Build history of the part. All positions in model axes, mm. A direction names the side the tool comes from. Round coordinates to 2 decimals unless told otherwise and drop trailing zeros. Write each loop counter-clockwise with the first axis right and the second up, starting at its lowest first coordinate (ties: lowest second). Pieces come first, ordered by that corner, then holes. Notation, with made-up numbers: (41.5, 34.5) -> (45.5, 34.5) arc R25 ccw to (45.5, 67.5) -> close; hole circle Ø11 at (-39, -12.5). An arc over 180 degrees is marked (long way). Return JSON: item names as keys, results as strings.
from build123d import *

# Parameters (mm, degrees)
F0_R     = 3
F1_DEPTH = 5
F0_R_2   = 1.6
F2_DEPTH = 2
F4_W     = 30
F4_H     = 20
F5_DEPTH = 2
F6_R     = 0.99999


# Not quite as in the source:
# - a fillet or chamfer is up to 0.001 mm smaller than in the source, because OpenCascade refuses the exact size


with BuildPart() as f1:
    # F0 (on Top) → F1 (new body)
    with BuildSketch(Plane.XY):
        with BuildLine():
            Line((-47.4, -10), (0, -10))
            ThreePointArc((0, -10), (10, 0), (0, 10))
            Line((0, 10), (-47.4, 10))
            ThreePointArc((-47.4, 10), (-57.4, 0), (-47.4, -10))
        make_face()
        with Locations((-47.4, 0)):
            Circle(F0_R, mode=Mode.SUBTRACT)
        Polygon((-6.5240580418, 0), (-3.2620290209, 5.65), (3.2620290209, 5.65), (6.5240580418, 0), (3.2620290209, -5.65), (-3.2620290209, -5.65), align=None, mode=Mode.SUBTRACT)
    extrude(amount=F1_DEPTH)

    # F0 (on Top) → F2 (join)
    with BuildSketch(Plane.XY):
        Polygon((3.2620290209, 5.65), (-3.2620290209, 5.65), (-6.5240580418, 0), (-3.2620290209, -5.65), (3.2620290209, -5.65), (6.5240580418, 0), align=None)
        Circle(F0_R_2, mode=Mode.SUBTRACT)
    extrude(amount=F2_DEPTH)

    # F4 (on face) → F5 (cut)
    with BuildSketch(Plane(origin=(0, 0, 0), x_dir=(1, 0, 0), z_dir=(0, 0, -1))):
        with Locations((-44.4, 0)):
            Rectangle(F4_W, F4_H)
    extrude(amount=-F5_DEPTH, mode=Mode.SUBTRACT)

    # F6 (radius 1 in the source; OpenCascade refuses exactly that, so slightly less here)
    f6_edges = [f1.edges().sort_by_distance(p)[0] for p in [
        (-29.4, 0, 2),
        (-29.4, 0, 0),
    ]]
    fillet(f6_edges, radius=F6_R)


solid = f1.part
Q1. Pin check, flat tips, straight feed: pin 1 Ø10 at (x, y) = (-42.5, -2) entering from -Z; pin 2 Ø0.9 at (x, z) = (1.5, 3.5) entering from +Y. Stop position of each tip, or through.
Verdict:
{"pin 1": "stops at z = 2", "pin 2": "stops at y = 9.94"}
Q2. Wall check: L1, parallel to X at y = 0, z = 2.95; L2, parallel to X at y = -1.5, z = 3.9; L3, parallel to Z at x = -31, y = 1.5. Give the ranges that are in metal, low to high.
Verdict:
{"L1": "x = -57.4 to -50.4, -44.4 to -6.52, 6.52 to 10", "L2": "x = -57.29 to -50, -44.8 to -5.66, 5.66 to 9.89", "L3": "z = 2 to 5"}
Q3. Two-plate mould, pull along X, no slides. Class faces 4 (the flat face through (0, -5.65, 3)), 5 (the flat face through (-19, -10, 2)), 6 (the cylindrical face through (10, 0, 2)): +X half, -X half, draft (parallel to the pull), parting line (faces both ways), or undercut.
Verdict:
{"face 4": "undercut", "face 5": "draft", "face 6": "+X half"}
Q4. Saw through at D-D on x = -38. List the corners of the cut face in (y, z).
Verdict:
{"outline": "(-10, 2) -> (10, 2) -> (10, 5) -> (-10, 5) -> close"}
Q5. Saw through at A-A on z = 3.05. List the corners of the cut face in (x, y), then the cut area to 3 significant figures.
Verdict:
{"outline": "(-47.4, -10) -> (0, -10) arc R10 ccw to (0, 10) -> (-47.4, 10) arc R10 ccw to start; hole circle Ø6 at (-47.4, 0); hole (-6.52, 0) -> (-3.26, -5.65) -> (3.26, -5.65) -> (6.52, 0) -> (3.26, 5.65) -> (-3.26, 5.65) -> close", "area": "1,120 mm²"}
Q6. 3-axis set-ups, long thin cutter, end or side, ignore diameter. For faces 1 (the flat face through (1.4, 1.3, 2)), 2 (the flat face through (-9, 0, 0)), 3 (the flat face through (-44, 0, 2)): which of +Z, -Z, +X, -X, +Y, -Y reach the whole face in a straight line?
Verdict:
{"face 1": "+Z", "face 2": "-Z, +X, -X, +Y, -Y", "face 3": "-Z, -X, +Y, -Y"}
